Check sheet for the modelled part. Datum: model origin and axes. Units: mm. A direction names the side the tool comes from. Round coordinates to 2 decimals unless told otherwise and drop trailing zeros. Write each loop counter-clockwise with the first axis right and the second up, starting at its lowest first coordinate (ties: lowest second). Pieces come first, ordered by that corner, then holes. Notation, with made-up numbers: M 27.25,89 L 34.25,89 A26 cw 34.25,117 Z; hole C 26.25,-20.5 d6. An arc over 180 degrees is marked long. Put each result on its own line as item: value.
```python
from build123d import *

# Parameters (mm, degrees)
BOSS_EXTRUDE1_DEPTH = 10
BOSS_EXTRUDE2_DEPTH = 1.5


with BuildPart() as part:
    # Sketch1 → Boss-Extrude1 (new body)
    with BuildSketch(Plane.XY):
        Polygon((0, 0), (20, -11.547005384), (21, -9.814954576), (0, 2.309401077), (-18.320508076, -8.267949192), (-17.320508076, -10), align=None)
    extrude(amount=BOSS_EXTRUDE1_DEPTH)

    # Sketch2 → Boss-Extrude2 (add)
    with BuildSketch(Plane.XY.offset(10)):
        Polygon((-18.320508076, -8.267949192), (0, 2.309401077), (21, -9.814954576), (20, -11.547005384), (14.226497308, -21.547005384), (-11.547005384, -20), (-17.320508076, -10), align=None)
    boss_extrude2 = extrude(amount=BOSS_EXTRUDE2_DEPTH)

    # Mirror1: Boss-Extrude2 across plane
    add(boss_extrude2.mirror(Plane(origin=(0, 0, 5), x_dir=(1, 0, 0), z_dir=(0, 0, -1))))


solid = part.part
```
1. Scan lines: probe 1 along Z at (x, y) = (-5, -14); probe 2 along X at (y, z) = (-3.5, 5.75); probe 3 along Y at (x, z) = (3.5, 0.5). Record each from-to range of solid material in increasing order.
Computed values:
probe 1: z = -1.5 to 0, 10 to 11.5
probe 2: x = -10.06 to -6.06, 6.06 to 10.06
probe 3: y = -2.02 to 0.29
2. Cross-section at B-B (y = -16.25). Enter the section's corners in (x, z).
Computed values:
outline: M -13.71,-1.5 L 17.28,-1.5 L 17.28,0 L -13.71,0 Z; M -13.71,10 L 17.28,10 L 17.28,11.5 L -13.71,11.5 Z
3. Release check for a two-part mould opening along Z. For faces 1 (the flat face through (-9.288, -3.053, 5.091)), 2 (the flat face through (-8.78, -5.07, 4.93)), 3 (the flat face through (2, -12, -1.5)), 4 (the flat face through (2, -13, 10)) record: +Z half, -Z half, draft (parallel to the pull), parting line (faces both ways), or undercut.
Computed values:
face 1: draft
face 2: undercut
face 3: -Z half
face 4: undercut
4. Cross-section at A-A (y = -2). Enter the section's corners in (x, z).
Computed values:
outline: M -7.46,-1.5 L 7.46,-1.5 L 7.46,11.5 L -7.46,11.5 Z; hole M -3.46,0 L 3.46,0 L 3.46,10 L -3.46,10 Z
5. Access from +Z, -Z, +X, -X, +Y, -Y to the whole of each face (thin tool, end or side, straight path). Record for faces 5 (the flat face through (9.86, -5.693, 4.93)), 6 (the flat face through (1.52, -20.784, 10.74)).
Computed values:
face 5: -Y
face 6: +Z, -Z, -X, -Y
6. Depth check by flat-ended pin: pin 1 Ø4 at (y, z) = (-3.5, 2.5) entering from -X; pin 2 Ø5 at (x, z) = (-7.5, 8.5) entering from +Y; pin 3 Ø5 at (y, z) = (-15, 9.5) entering from +X; pin 4 Ø3 at (y, z) = (-14.5, 6) entering from +X. Enter the tip coordinate at first touch or a pass-through.
Computed values:
pin 1: stops at x = -13.53
pin 2: stops at y = -0.58
pin 3: stops at x = 19.42
pin 4: passes through
7. Cross-section at D-D (x = 4). Enter the section's corners in (y, z).
Computed values:
outline: M -20.93,-1.5 L 0,-1.5 L 0,11.5 L -20.93,11.5 L -20.93,10 L -2.31,10 L -2.31,0 L -20.93,0 Z
8. Cross-section at C-C (z = 1.75). Enter the section's corners in (x, y), then the cut area to 3 significant figures.
Computed values:
outline: M -18.32,-8.27 L -17.32,-10 L 0,0 L 20,-11.55 L 21,-9.81 L 0,2.31 Z
area: 88.5 mm2
